Work out the finished part from the listing and answer in its coordinate system (mm). A direction names the side the tool comes from. Coordinates: 2 decimals unless noted, no trailing zeros. Write each loop counter-clockwise with the first axis right and the second up, starting at its lowest first coordinate (ties: lowest second). Pieces come first, ordered by that corner, then holes. Notation, with made-up numbers: (39.5, 30) - (64.5, 30) arc R16 ccw to (64.5, 52) - close; hole circle Ø10 at (-20, -10). An arc over 180 degrees is marked (long way). Use CSV: the item, a comma, the result in double quotes. Start each with the question number.
from build123d import *

# Parameters (mm, degrees)
SKETCH_1_R      = 2.5
EXTRUDE_1_DEPTH = 47
EXTRUDE_START   = 47
SKETCH_2_R      = 4
EXTRUDE_2_DEPTH = 49
EXTRUDE_START_2 = 96
SKETCH_3_R      = 5
EXTRUDE_3_DEPTH = 3.5
EXTRUDE_START_3 = 99.5
SKETCH_4_R      = 4
EXTRUDE_4_DEPTH = 18
EXTRUDE_START_4 = 2.2
EXTRUDE_5_DEPTH = 3
CHAMFER_1_SIZE  = 0.25
CHAMFER_2_SIZE  = 0.1


with BuildPart() as part:
    # 草图1 → 凸台-拉伸1 (new body)
    with BuildSketch(Plane(origin=(0, 0, 0), x_dir=(1, 0, 0), z_dir=(0, 1, 0))):
        with Locations(Location((0, 0, 0), (0, 0, 270))):
            Circle(SKETCH_1_R)
    extrude(amount=EXTRUDE_1_DEPTH)

    # 草图2 → 凸台-拉伸2 (add)
    with BuildSketch(Plane(origin=(0, 0, 0), x_dir=(1, 0, 0), z_dir=(0, 1, 0)).offset(EXTRUDE_START)):
        with Locations(Location((0, 0, 0), (0, 0, 270))):
            Circle(SKETCH_2_R)
    extrude(amount=EXTRUDE_2_DEPTH)

    # 草图3 → 凸台-拉伸3 (add)
    with BuildSketch(Plane(origin=(0, 0, 0), x_dir=(1, 0, 0), z_dir=(0, 1, 0)).offset(EXTRUDE_START_2)):
        with Locations(Location((0, 0, 0), (0, 0, 270))):
            Circle(SKETCH_3_R)
    extrude(amount=EXTRUDE_3_DEPTH)

    # 草图4 → 凸台-拉伸4 (add)
    with BuildSketch(Plane(origin=(0, 0, 0), x_dir=(1, 0, 0), z_dir=(0, 1, 0)).offset(EXTRUDE_START_3)):
        with Locations(Location((0, 0, 0), (0, 0, 270))):
            Circle(SKETCH_4_R)
    extrude(amount=EXTRUDE_4_DEPTH)

    # 草图9 → M3 螺纹孔1 (revolve, cut)
    with BuildSketch(Plane(origin=(0, 117.5, 0), x_dir=(0, 0, 1), z_dir=(1, 0, 0))):
        Polygon((0, 0), (0, 10.751075774), (1.25, 10), (1.25, 0), align=None)
    revolve(axis=Axis((0, 123.85, 0), (0, -1, 0)), mode=Mode.SUBTRACT)

    # 草图11 → 凸台-拉伸5 (add)
    with BuildSketch(Plane.XY.offset(EXTRUDE_START_4)):
        with BuildLine():
            Line((-1.5, 103), (-1.5, 114))
            ThreePointArc((-1.5, 114), (0, 115.5), (1.5, 114))
            Line((1.5, 114), (1.5, 103))
            ThreePointArc((1.5, 103), (0, 101.5), (-1.5, 103))
        make_face()
    extrude(amount=EXTRUDE_5_DEPTH)

    # 倒角1
    chamfer_1_edges = [part.edges().sort_by_distance(p)[0] for p in [
        (0, 117.5, -4),
        (0, 0, -2.5),
    ]]
    chamfer(chamfer_1_edges, length=CHAMFER_1_SIZE)

    # 倒角2
    chamfer_2_edges = [part.edges().sort_by_distance(p)[0] for p in [
        (0, 101.5, 5.2),
        (1.5, 108.5, 5.2),
        (0, 115.5, 5.2),
        (-1.5, 108.5, 5.2),
    ]]
    chamfer(chamfer_2_edges, length=CHAMFER_2_SIZE)


solid = part.part
Item 1: Straight lines are drawn through the part: probe 1 along X at (y, z) = (114, 0); probe 2 along Y at (x, z) = (4.25, -1); probe 3 along Y at (x, z) = (-0.25, 2.25). For each, find the intervals that lie inside material, in ascending order. Write a range as [from, to].
Item 2: Determine the mould class of faces 1 (the face through (0.21, 106.88, -0.05)), 2 (the face through (2, 47, 2)), 3 (the face through (-4.88, 97.73, -1.08)) for opening direction X: +X half, -X half, draft (parallel to the pull), parting line (faces both ways), or undercut.
Item 3: A cutting plane is placed at A-A (y = 50.5). Determine the outline of the cut face in (x, z).
Item 4: Which of the six approach directions +Z, -Z, +X, -X, +Y, -Y give full straight-line access (tool end or side, diameter ignored) to faces 4 (the face through (-3.905, 71.157, -0.867)), 5 (the face through (0, 109, 5.2)), 6 (the face through (1.22, 112.57, -0.27))?
Item 5: Each of these flat-tipped pins is pushed along its axis until it touches: pin 1 (2 mm diameter, centred on x = -2.5, z = 4, fed in from -Y); pin 2 (6 mm diameter, centred on x = 0.5, y = 32, fed in from -Z); pin 3 (1.5 mm diameter, centred on y = 110, z = 4.5, fed in from -X). Where does it stop, or does it pass through?
Calculated:
1,probe 1,"x = [-4, -1.25], [1.25, 4]"
1,probe 2,"y = [96, 99.5]"
1,probe 3,"y = [0.01, 117.5]"
2,face 1,"undercut"
2,face 2,"draft"
2,face 3,"parting line"
3,outline,"circle Ø8 at (0, 0)"
4,face 4,"-Y"
4,face 5,"+Z, +X, -X, +Y, -Y"
4,face 6,"+Y"
5,pin 1,"stops at y = 47"
5,pin 2,"stops at z = -2.5"
5,pin 3,"stops at x = -1.5"
